from build123d import *

# Parameters (mm, degrees)
DODANIE_WYCI_GNI_CIE1_DEPTH = 5
SZKIC3_R                    = 2
WYTNIJ_WYCI_GNI_CIE1_DEPTH  = 5
SZKIC4_W                    = 4
SZKIC4_H                    = 10
WYTNIJ_WYCI_GNI_CIE2_DEPTH  = 5
ZAOKR_GLENIE1_R             = 3
ZAOKR_GLENIE2_R             = 2
SZKIC5_W                    = 13
SZKIC5_H                    = 25
DODANIE_WYCI_GNI_CIE2_DEPTH = 5
SFAZOWANIE1_SIZE            = 5
WYTNIJ_WYCI_GNI_CIE3_REACH  = 232.76
SZKIC6_R                    = 1.75


with BuildPart() as part:
    # Szkic2 → Dodanie-wyciągnięcie1 (new body)
    with BuildSketch(Plane.XY):
        Polygon((0, 0), (30, 0), (30, 30), (85, 90), (115, 90), (170, 30), (170, 0), (200, 0), (200, 30), (120, 115), (80, 115), (0, 30), align=None)
    extrude(amount=DODANIE_WYCI_GNI_CIE1_DEPTH)

    # Szkic3 → Wytnij-wyciągnięcie1 (cut)
    with BuildSketch(Plane.XY.offset(5)):
        with Locations((15, 15)):
            Circle(SZKIC3_R)
        with Locations((185, 15)):
            Circle(SZKIC3_R)
    extrude(amount=-WYTNIJ_WYCI_GNI_CIE1_DEPTH, mode=Mode.SUBTRACT)

    # Szkic4 → Wytnij-wyciągnięcie2 (cut)
    with BuildSketch(Plane.XY.offset(5)):
        with Locations((100, 98)):
            Rectangle(SZKIC4_W, SZKIC4_H)
    extrude(amount=-WYTNIJ_WYCI_GNI_CIE2_DEPTH, mode=Mode.SUBTRACT)

    # Zaokrąglenie1
    zaokr_glenie1_edges = [part.edges().sort_by_distance(p)[0] for p in [
        (0, 30, 2.5),
        (80, 115, 2.5),
        (120, 115, 2.5),
        (200, 30, 2.5),
        (200, 0, 2.5),
        (170, 0, 2.5),
        (30, 0, 2.5),
        (0, 0, 2.5),
    ]]
    fillet(zaokr_glenie1_edges, radius=ZAOKR_GLENIE1_R)

    # Zaokrąglenie2
    zaokr_glenie2_edges = [part.edges().sort_by_distance(p)[0] for p in [
        (98, 103, 2.5),
        (102, 103, 2.5),
        (102, 93, 2.5),
        (98, 93, 2.5),
    ]]
    fillet(zaokr_glenie2_edges, radius=ZAOKR_GLENIE2_R - 0.0001)  # a hair under: the kernel refuses the full size

    # Szkic5 → Dodanie-wyciągnięcie2 (add)
    with BuildSketch(Plane.XY.offset(5)):
        with Locations((113.5, 102.5)):
            Rectangle(SZKIC5_W, SZKIC5_H)
        with Locations((86.5, 102.5)):
            Rectangle(SZKIC5_W, SZKIC5_H)
    extrude(amount=DODANIE_WYCI_GNI_CIE2_DEPTH)

    # Sfazowanie1
    sfazowanie1_edges = [part.edges().sort_by_distance(p)[0] for p in [
        (80, 102.5, 10),
        (120, 102.5, 10),
    ]]
    chamfer(sfazowanie1_edges, length=SFAZOWANIE1_SIZE - 0.0001)  # a hair under: the kernel refuses the full size

    # Szkic6 → Wytnij-wyciągnięcie3 (cut, up to next)
    with BuildSketch(Plane.XY.offset(5), mode=Mode.PRIVATE) as wytnij_wyci_gni_cie3_sk1:
        with Locations((74.778017415, 83.288424616)):
            Circle(SZKIC6_R)
    wytnij_wyci_gni_cie3_tool1 = extrude(wytnij_wyci_gni_cie3_sk1.sketch, amount=-WYTNIJ_WYCI_GNI_CIE3_REACH, mode=Mode.PRIVATE) & part.part
    # Szkic6 → Wytnij-wyciągnięcie3 (cut, up to next)
    with BuildSketch(Plane.XY.offset(5), mode=Mode.PRIVATE) as wytnij_wyci_gni_cie3_sk2:
        with Locations((34.234539704, 39.059176204)):
            Circle(SZKIC6_R)
    wytnij_wyci_gni_cie3_tool2 = extrude(wytnij_wyci_gni_cie3_sk2.sketch, amount=-WYTNIJ_WYCI_GNI_CIE3_REACH, mode=Mode.PRIVATE) & part.part
    # Szkic6 → Wytnij-wyciągnięcie3 (cut, up to next)
    with BuildSketch(Plane.XY.offset(5), mode=Mode.PRIVATE) as wytnij_wyci_gni_cie3_sk3:
        with Locations((54.50627856, 61.17380041)):
            Circle(SZKIC6_R)
    wytnij_wyci_gni_cie3_tool3 = extrude(wytnij_wyci_gni_cie3_sk3.sketch, amount=-WYTNIJ_WYCI_GNI_CIE3_REACH, mode=Mode.PRIVATE) & part.part
    add(wytnij_wyci_gni_cie3_tool1.solids().sort_by_distance((74.778017, 83.288425, 5))[0], mode=Mode.SUBTRACT)
    add(wytnij_wyci_gni_cie3_tool2.solids().sort_by_distance((34.23454, 39.059176, 5))[0], mode=Mode.SUBTRACT)
    add(wytnij_wyci_gni_cie3_tool3.solids().sort_by_distance((54.506279, 61.1738, 5))[0], mode=Mode.SUBTRACT)


solid = part.part
Geometry: final body of the model. Coordinates: model frame, mm. A direction names the side the tool comes from. Round coordinates to 2 decimals unless told otherwise and drop trailing zeros. Order: outer loops, then holes, each group sorted by start corner. A loop starts at its lowest first (then second) coordinate and runs counter-clockwise, first axis right, second up.
Q1. Mould query, pull axis Y, two halves, no side actions, for faces 1 (the face through (15, 0, 2)), 2 (the face through (102, 98, 3)), 3 (the face through (0, 16, 2)). Classes: released by +Y, released by -Y, zero draft, split by the parting line, or undercut.
Result sheet:
face 1: released by -Y
face 2: undercut
face 3: zero draft
Q2. Material intervals for probe 1 along X at (y, z) = (56, 2.25); probe 2 along X at (y, z) = (73.5, 2) (3 decimals); probe 3 along Y at (x, z) = (86, 5), sorted ascending.
Result sheet:
probe 1: x = 24.47 to 53.83, 146.17 to 175.53
probe 2: x = 40.941 to 69.875, 130.125 to 159.059
probe 3: y = 90 to 115
Q3. Section B-B, the plane z = 7. Output: boundary loops of the cut face in (x, y).
Result sheet:
outline: (82, 90) - (93, 90) - (93, 115) - (82, 115) - close; (107, 90) - (118, 90) - (118, 115) - (107, 115) - close
Q4. Access query for faces 4 (the face through (30, 16, 2)), 5 (the face through (98, 98, 3)), 6 (the face through (107, 102, 7)), 7 (the face through (118, 102, 7)), 8 (the face through (82, 102, 7)). Directions: +Z, -Z, +X, -X, +Y, -Y. A direction counts if a zero-diameter tool reaches every point of the face in a straight line with its end or side. Return the directions, or none.
Result sheet:
face 4: +Z, -Z, -Y
face 5: +Z, -Z
face 6: +Z, +Y, -Y
face 7: +Z, +X, +Y, -Y
face 8: +Z, -X, +Y, -Y
Q5. Section D-D, the plane x = 104. Output: boundary loops of the cut face in (y, z), and give its area (3 significant figures).
Result sheet:
outline: (90, 0) - (115, 0) - (115, 5) - (90, 5) - close
area: 125 mm2
Q6. Pin query (flat end, axial travel): pin 1 (5 mm diameter, centred on x = 156, z = 2.5, fed in from -Y); pin 2 (5.5 mm diameter, centred on x = 34.23, y = 39.06, fed in from +Z); pin 3 (5 mm diameter, centred on y = 93.5, z = 2, fed in from +X). Return the tip coordinate at first contact, or that it passes through.
Result sheet:
pin 1: stops at y = 42.55
pin 2: stops at z = 5
pin 3: stops at x = 142.59
Q7. Section A-A, the plane y = 15. Output: boundary loops of the cut face in (x, z).
Result sheet:
outline: (0, 0) - (13, 0) - (13, 5) - (0, 5) - close; (17, 0) - (30, 0) - (30, 5) - (17, 5) - close; (170, 0) - (183, 0) - (183, 5) - (170, 5) - close; (187, 0) - (200, 0) - (200, 5) - (187, 5) - close
Q8. Section C-C, the plane y = 87.5. Output: boundary loops of the cut face in (x, z).
Result sheet:
outline: (54.12, 0) - (82.71, 0) - (82.71, 5) - (54.12, 5) - close; (117.29, 0) - (145.88, 0) - (145.88, 5) - (117.29, 5) - close
